Check sheet for the modelled part. Datum: model origin and axes. Units: mm. A direction names the side the tool comes from. Coordinates: 2 decimals unless noted, no trailing zeros. Loops run counter-clockwise (first coordinate to the right, second up) from the corner with the lowest first, then second, coordinate; pieces in that order, holes last. Notation, with made-up numbers: M 20.25,-14.75 L 59.25,-14.75 A14 ccw 59.25,-7.75 Z; hole C -34.75,21 d7. An arc over 180 degrees is marked long. Use CSV: the item, a comma, the result in double quotes. Start each with the question number.
(1) Draft check along Y on faces 1 (the flat face through (-81, 22, 83)), 2 (the flat face through (-80, 39.5, 62)), 3 (the flat face through (-86, 0, 84)). Enter one of: pulls with the +Y half, pulls with the -Y half, needs draft (parallel to the pull), parting line crosses it, or undercut.
(2) Section check A-A on x = -32. Record the cut outline in (y, z).
(3) Set-up check for faces 4 (the flat face through (-49, 39, 56)), 5 (the flat face through (-10, 65, 16)), 6 (the flat face through (-105, 45, 62)): record each of +Z, -Z, +X, -X, +Y, -Y from which the full face is reachable in a straight line by a thin tool's end or side.
(4) Go/stop test with flat-tipped pins: pin 1 Ø13 at (x, y) = (-114.5, 13.5) entering from +Z; pin 2 Ø4 at (y, z) = (57.5, 16.5) entering from -X; pin 3 Ø25 at (x, z) = (-82.5, 64) entering from +Y. Record where each tip stops, or that it passes through.
(5) Section check D-D on z = 37.5. Record the cut outline in (x, y).
(6) Scan lines: line 1 (Z direction, x = -80, y = 35.05); line 2 (Y direction, x = -45, z = 84.5); line 3 (X direction, y = 102, z = 43). Record each from-to range of solid material in increasing order.
(7) Section check B-B on z = 72. Record the cut outline in (x, y), and give its area (3 significant figures).
(8) Section check C-C on y = 14. Record the cut outline in (x, z).
from build123d import *

# Parameters (mm, degrees)
SKETCH1_W                = 160
SKETCH1_H                = 49.5
BOSS_EXTRUDE1_DEPTH      = 89
BOSS_EXTRUDE2_DEPTH      = 16
SKETCH2_W                = 50
SKETCH2_H                = 54
SKETCH2_R                = 7.5
CUT_EXTRUDE1_DEPTH       = 10
SHELL2_T                 = -6
SKETCH1_4_R              = 32
SKETCH1_4_R_2            = 17.5
BOSS_EXTRUDE3_DEPTH      = 92.4
BOSS_EXTRUDE4_REACH      = 205.378
BOSS_EXTRUDE4_END_RADIUS = 32
SKETCH2_8_R              = 7.5
CUT_EXTRUDE4_DEPTH       = 204.378366598


with BuildPart() as part:
    # Sketch1 → Boss-Extrude1 (new body)
    with BuildSketch(Plane.XY):
        with Locations((-80, 24.75)):
            Rectangle(SKETCH1_W, SKETCH1_H)
    extrude(amount=BOSS_EXTRUDE1_DEPTH)

    # Sketch2 → Cut-Extrude1 (cut)
    with BuildSketch(Plane(origin=(0, 49.5, 0), x_dir=(1, 0, 0), z_dir=(0, 1, 0))):
        with Locations((-80, -62)):
            Rectangle(SKETCH2_W, SKETCH2_H)
        with Locations(Location((-80, -72, 0), (0, 0, 180))):
            Circle(SKETCH2_R, mode=Mode.SUBTRACT)
        with Locations(Location((-80, -47, 0), (0, 0, 180))):
            Circle(SKETCH2_R, mode=Mode.SUBTRACT)
    extrude(amount=-CUT_EXTRUDE1_DEPTH, mode=Mode.SUBTRACT)

    # Shell2
    shell2_openings = [part.faces().sort_by_distance(p)[0] for p in [
        (-80, 0, 44.5),
    ]]
    offset(amount=SHELL2_T, openings=shell2_openings, kind=Kind.INTERSECTION)

    # Boss-Extrude4: up to this cylinder (the profile starts outside it)
    boss_extrude4_end = Plane(origin=(-32, 102.5, 38.177591), z_dir=(0, 0, -1)) * Cylinder(BOSS_EXTRUDE4_END_RADIUS, 475.756, mode=Mode.PRIVATE)
    # Sketch2<6> → Boss-Extrude4 (add, up to the surface)
    with BuildSketch(Plane(origin=(0, 49.5, 0), x_dir=(1, 0, 0), z_dir=(0, 1, 0)), mode=Mode.PRIVATE) as boss_extrude4_sk1:
        with BuildLine():
            Line((-40, -16), (-24, -16))
            Line((-24, -16), (-24, -54))
            ThreePointArc((-24, -54), (-32, -62), (-40, -54))
            Line((-40, -54), (-40, -16))
        make_face()
    boss_extrude4_tool1 = extrude(boss_extrude4_sk1.sketch, amount=BOSS_EXTRUDE4_REACH, mode=Mode.PRIVATE) - boss_extrude4_end
    add(boss_extrude4_tool1.solids().sort_by_distance((-32, 49.5, 38.177591))[0])

    # Sketch2<8> → Cut-Extrude4 (cut, through all)
    with BuildSketch(Plane(origin=(0, 49.5, 0), x_dir=(1, 0, 0), z_dir=(0, 1, 0))):
        with Locations(Location((-80, -47, 0), (0, 0, 180))):
            Circle(SKETCH2_8_R)
        with Locations(Location((-80, -72, 0), (0, 0, 180))):
            Circle(SKETCH2_8_R)
    extrude(amount=-CUT_EXTRUDE4_DEPTH, mode=Mode.SUBTRACT)


with BuildPart() as body_2:
    # Sketch1<3> → Boss-Extrude2 (new body)
    with BuildSketch(Plane.XY):
        with BuildLine():
            Line((-160, 49.5), (0, 49.5))
            Line((0, 49.5), (0, 102.5))
            ThreePointArc((0, 102.5), (-47.127064471, 74.301207109), (-49.698245031, 129.160309879))
            Line((-49.698245031, 129.160309879), (-154.636841887, 59.497616205))
            ThreePointArc((-154.636841887, 59.497616205), (-158.574547334, 55.172649177), (-160, 49.5))
        make_face()
    extrude(amount=BOSS_EXTRUDE2_DEPTH)


with BuildPart() as body_3:
    # Sketch1<4> → Boss-Extrude3 (new body)
    with BuildSketch(Plane.XY):
        with Locations((-32, 102.5)):
            Circle(SKETCH1_4_R)
        with Locations((-32, 102.5)):
            Circle(SKETCH1_4_R_2, mode=Mode.SUBTRACT)
    extrude(amount=BOSS_EXTRUDE3_DEPTH)

    # Combine1: union part, body 2
    add(part.part)
    add(body_2.part)


solid = body_3.part
Outcome:
1,face 1,"needs draft"
1,face 2,"undercut"
1,face 3,"pulls with the -Y half"
2,outline,"M 0,0 L 85,0 L 85,92.4 L 70.5,92.4 L 70.5,62 L 49.5,62 L 49.5,89 L 0,89 L 0,83 L 43.5,83 L 43.5,6 L 0,6 Z; M 120,0 L 134.5,0 L 134.5,92.4 L 120,92.4 Z"
3,face 4,"-Y"
3,face 5,"+Z, +X"
3,face 6,"+Z, +Y"
4,pin 1,"stops at z = 89"
4,pin 2,"stops at x = -158.36"
4,pin 3,"stops at y = 39.5"
5,outline,"M -160,0 L -154,0 L -154,43.5 L -111,43.5 L -111,33.5 L -49,33.5 L -49,43.5 L -6,43.5 L -6,0 L 0,0 L 0,49.5 L -24,49.5 L -24,71.52 A32 ccw long -40,71.52 L -40,49.5 L -55,49.5 L -55,39.5 L -105,39.5 L -105,49.5 L -160,49.5 Z; hole C -32,102.5 d35"
6,line 1,"z = 0 to 6, 29 to 39.5, 54.5 to 64.5, 79.5 to 89"
6,line 2,"y = 0 to 49.5, 73.26 to 90.78, 114.22 to 131.74"
6,line 3,"x = -64 to -49.49, -14.51 to 0"
7,outline,"M -160,0 L -154,0 L -154,43.5 L -111,43.5 L -111,33.5 L -87.5,33.5 L -87.5,39.5 L -105,39.5 L -105,49.5 L -160,49.5 Z; M -72.5,33.5 L -49,33.5 L -49,43.5 L -6,43.5 L -6,0 L 0,0 L 0,49.5 L -55,49.5 L -55,39.5 L -72.5,39.5 Z; C -32,102.5 d64; hole C -32,102.5 d35"
7,area,"3,770 mm²"
8,outline,"M -160,0 L 0,0 L 0,89 L -160,89 Z; hole M -154,6 L -6,6 L -6,83 L -154,83 Z"
